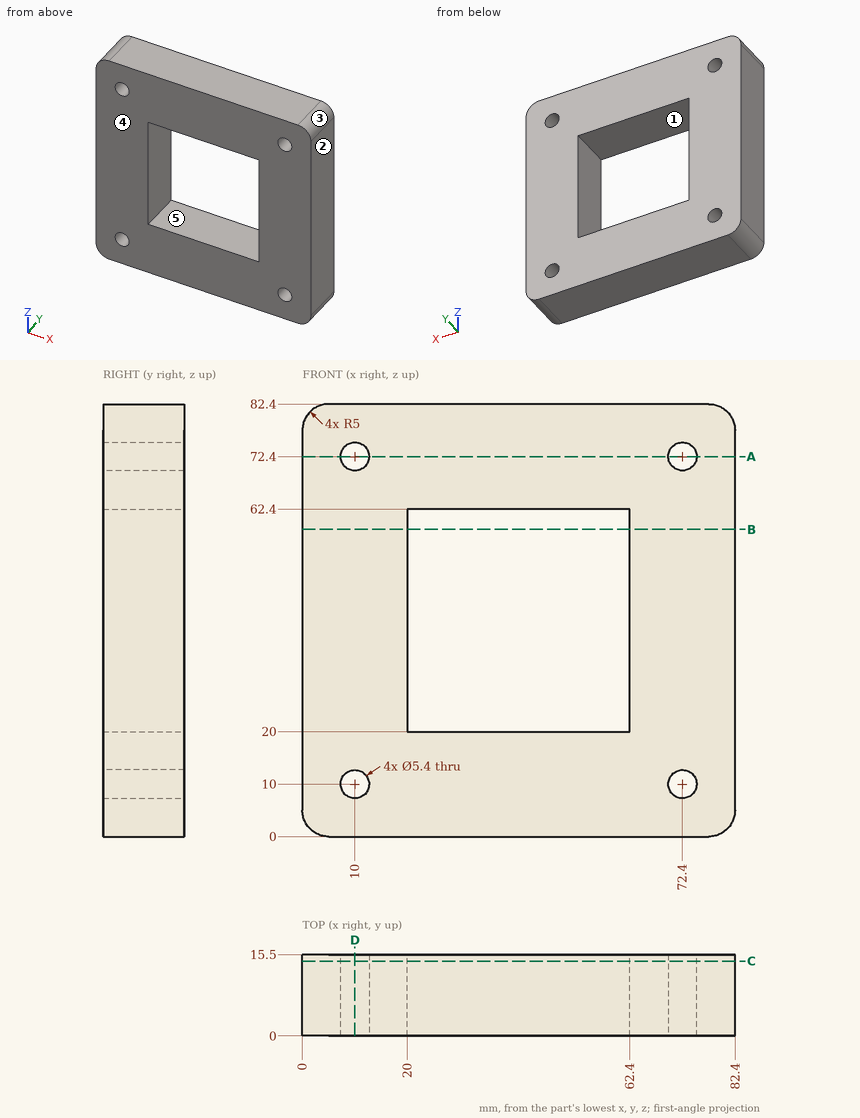
The figure shows three views and two pictorial views of one solid part (mm, origin at its lowest corner). Answer the questions. A direction names the side the tool comes from. Coordinates: 2 decimals unless noted, no trailing zeros. Loops run counter-clockwise (first coordinate to the right, second up) from the corner with the lowest first, then second, coordinate; pieces in that order, holes last. Notation, with made-up numbers: (48, -25) -> (94, -25) arc R19 ccw to (94, 4) -> close; hole circle Ø1 at (71, -39.5). An arc over 180 degrees is marked (long way). Use one line per item in the form item = value. Start each with the question number.
Item 1: The mould has two halves that part along X. Classify the marked faces 3, 4 and 5: released by +X, released by -X, zero draft, split by the parting line, or undercut.
Item 2: A tool of negligible diameter and unlimited length cuts with its end or side. For the marked faces 1 and 2, from which of +Z, -Z, +X, -X, +Y, -Y can it reach the whole face along a straight path? Write none if from no direction.
Item 3: The part is cut by section D-D on x = 10. Determine the outline of the cut face in (y, z).
Item 4: Consider L1, parallel to X at y = 12.5, z = 72.4; L2, parallel to Z at x = 34.5, y = 6. Determine where each line is inside the solid, lowest interval first. Write a range as [from, to].
Item 5: The part is cut by section A-A on z = 72.4. Determine the outline of the cut face in (x, y), then the cut area to 3 significant figures.
Item 6: The part is cut by section C-C on y = 14.25. Determine the outline of the cut face in (x, z).
Item 7: The part is cut by section B-B on z = 58.5. Determine the outline of the cut face in (x, y), then the cut area to 3 significant figures.
Item 8: A flat-ended cylindrical pin translates along its axis: pin 1 Ø4.5 at (x, z) = (10, 72.4) entering from -Y. Find the tip coordinate at first contact, or state that the pin passes through.
Answer key:
q1.face_3 = released by +X
q1.face_4 = zero draft
q1.face_5 = undercut
q2.face_1 = +Y, -Y
q2.face_2 = +Z, -Z, +X, +Y, -Y
q3.outline = (0, 0) -> (15.5, 0) -> (15.5, 7.3) -> (0, 7.3) -> close; (0, 12.7) -> (15.5, 12.7) -> (15.5, 69.7) -> (0, 69.7) -> close; (0, 75.1) -> (15.5, 75.1) -> (15.5, 82.4) -> (0, 82.4) -> close
q4.L1 = [0, 7.3], [12.7, 69.7], [75.1, 82.4]
q4.L2 = [0, 20], [62.4, 82.4]
q5.outline = (0, 0) -> (7.3, 0) -> (7.3, 15.5) -> (0, 15.5) -> close; (12.7, 0) -> (69.7, 0) -> (69.7, 15.5) -> (12.7, 15.5) -> close; (75.1, 0) -> (82.4, 0) -> (82.4, 15.5) -> (75.1, 15.5) -> close
q5.area = 1,110 mm2
q6.outline = (0, 5) arc R5 ccw to (5, 0) -> (77.4, 0) arc R5 ccw to (82.4, 5) -> (82.4, 77.4) arc R5 ccw to (77.4, 82.4) -> (5, 82.4) arc R5 ccw to (0, 77.4) -> close; hole circle Ø5.4 at (10, 10); hole circle Ø5.4 at (10, 72.4); hole (20, 20) -> (62.4, 20) -> (62.4, 62.4) -> (20, 62.4) -> close; hole circle Ø5.4 at (72.4, 10); hole circle Ø5.4 at (72.4, 72.4)
q7.outline = (0, 0) -> (20, 0) -> (20, 15.5) -> (0, 15.5) -> close; (62.4, 0) -> (82.4, 0) -> (82.4, 15.5) -> (62.4, 15.5) -> close
q7.area = 620 mm2
q8.pin_1 = through
